Autodesk Inventor part; units mm, degrees
ref_plane "YZ Plane" through (0, 0, 0) normal (1, 0, 0) x (0, 1, 0)
ref_plane "XZ Plane" through (0, 0, 0) normal (0, 1, 0) x (-1, 0, 0)
ref_plane "XY Plane" through (0, 0, 0) normal (0, 0, 1) x (1, 0, 0)
sketch "Sketch1" plane through (0, 0, 0) normal (0, 1, 0) x (-1, 0, 0)
  line L0 (0, 0) -> (203.2, 0)
  line L1 (203.2, 0) -> (203.2, -101.6)
  line L2 (203.2, -101.6) -> (0, -101.6)
  line L3 (0, -101.6) -> (0, 0)
  dimension "d0" = 203.2
  dimension "d1" = 101.6
extrude "Extrusion1" add sketch "Sketch1" along normal blind 1.5875
sketch "Sketch2" plane through (0, 1.5875, 0) normal (0, 1, 0) x (1, 0, 0)
  circle A0 centre (-30.9372, 67.945) radius 12.7
  line L0 (0, 0) -> (0, 101.6)
  line L1 (-203.2, 0) -> (0, 0)
  dimension "d4" = 25.4
  dimension "d5" = 30.9372
  dimension "d6" = 67.945
extrude "Extrusion2" cut sketch "Sketch2" against normal blind 25.4
properties part number "TSV-Panel"
Design review of the part built by this model. Coordinates are the model's own, in mm. Round coordinates to 2 decimals unless told otherwise and drop trailing zeros. Write each loop counter-clockwise with the first axis right and the second up, starting at its lowest first coordinate (ties: lowest second). Pieces come first, ordered by that corner, then holes. Notation, with made-up numbers: M 0,37 L 39,37 A20 ccw 39,59 Z; hole C 52,-2.5 d7. An arc over 180 degrees is marked long. One line per item, written item: value. Start each with the question number.
1. Clearance check with a flat-ended pin moving along its axis: P1, Ø8, axis at x = -107.5, z = -31.5, coming from the -Y side. State where the tip first meets the part, or that it passes through.
2. Draft analysis for pull direction Z (two halves, no side actions). For faces 1 (the face through (-25.077, 0.805, -56.678)), 2 (the face through (-100, 0, -50)), state which applies: pulls with the +Z half, pulls with the -Z half, needs draft (parallel to the pull), parting line crosses it, or undercut.
3. Take a section at B-B on x = -36.5. State the section outline as (y, z) points.
4. To check wall thickness, follow probe 1 along X at (y, z) = (1.5, -68); probe 2 along X at (y, z) = (1.2, -75); probe 3 along Z at (x, y) = (-20, 0.75). State the ranges of each line that lie inside material, in increasing order. Write a range as from..to.
5. Take a section at C-C on y = 0.9. State the section outline as (x, z) points (3 decimals), then the cut area to 3 significant figures.
6. Take a section at A-A on z = -77. State the section outline as (x, y) points, then the cut area to 3 significant figures.
Computed:
1. P1: stops at y = 0
2. face 1: undercut
2. face 2: needs draft
3. outline: M 0,-101.6 L 1.59,-101.6 L 1.59,-79.36 L 0,-79.36 Z; M 0,-56.53 L 1.59,-56.53 L 1.59,0 L 0,0 Z
4. probe 1: x = -203.2..-43.64, -18.24..0
4. probe 2: x = -203.2..-41.5, -20.38..0
4. probe 3: z = -101.6..-74.4, -61.49..0
5. outline: M -203.2,-101.6 L 0,-101.6 L 0,0 L -203.2,0 Z; hole C -30.937,-67.945 d25.4
5. area: 20,100 mm²
6. outline: M -203.2,0 L -39.84,0 L -39.84,1.59 L -203.2,1.59 Z; M -22.03,0 L 0,0 L 0,1.59 L -22.03,1.59 Z
6. area: 294 mm²
